from build123d import *

# Parameters (mm, degrees)
PAD_DEPTH         = 10
ARRAY001_COUNT    = 4
CYLINDER021_R     = 12
CYLINDER021_DEPTH = 124
CYLINDER022_R     = 22
CYLINDER022_DEPTH = 5
FILLET004_R       = 1
CYLINDER020_R     = 14
CYLINDER020_DEPTH = 124
FILLET001_R       = 0.6
FILLET002_R       = 1


with BuildPart() as long_hole_array:
    # Sketch → Pad (new body)
    with BuildSketch(Plane.XY):
        with BuildLine():
            ThreePointArc((-18.36954, -4), (-13.293607, -13.293607), (-4, -18.36954))
            ThreePointArc((-4, -18.36954), (-2.147351, -16.516891), (-4, -14.664242))
            ThreePointArc((-14.664242, -4), (-10.748023, -10.748023), (-4, -14.664242))
            ThreePointArc((-14.664242, -4), (-16.516891, -2.147351), (-18.36954, -4))
        make_face()
    extrude(amount=PAD_DEPTH)

    # Array001: long hole array ×4 about axis
    array001_axis = Axis((0, 0, 0), (0, 0, 1))


with BuildPart() as long_hole_array_1:
    add(long_hole_array.part)
    for i in range(1, ARRAY001_COUNT):
        add(long_hole_array.part.rotate(array001_axis, i * 360 / ARRAY001_COUNT))


with BuildPart() as top_hole_fusion:
    # Cylinder021 → Cylinder021 (new body)
    with BuildSketch(Plane.XY):
        Circle(CYLINDER021_R)
    extrude(amount=CYLINDER021_DEPTH)

    # Fusion004: union long hole array
    add(long_hole_array_1.part)


with BuildPart() as top_bottom_connector_fillet:
    # Cylinder022 → Cylinder022 (new body)
    with BuildSketch(Plane.XY):
        Circle(CYLINDER022_R)
    extrude(amount=CYLINDER022_DEPTH)

    # Fillet004
    fillet004_edges = [top_bottom_connector_fillet.edges().sort_by_distance(p)[0] for p in [
        (-22, 0, 5),
        (-22, 0, 0),
    ]]
    fillet(fillet004_edges, radius=FILLET004_R)


with BuildPart() as top_tube_cut_fillet:
    # Cylinder020 → Cylinder020 (new body)
    with BuildSketch(Plane.XY):
        Circle(CYLINDER020_R)
    extrude(amount=CYLINDER020_DEPTH)

    # Fillet001
    fillet001_edges = [top_tube_cut_fillet.edges().sort_by_distance(p)[0] for p in [
        (-14, 0, 124),
    ]]
    fillet(fillet001_edges, radius=FILLET001_R)

    # Fusion: union top bottom connector fillet
    add(top_bottom_connector_fillet.part)

    # Cut: cut top hole fusion
    add(top_hole_fusion.part, mode=Mode.SUBTRACT)

    # Fillet002
    fillet002_edges = [top_tube_cut_fillet.edges().sort_by_distance(p)[0] for p in [
        (-12, 0, 124),
    ]]
    fillet(fillet002_edges, radius=FILLET002_R)


solid = top_tube_cut_fillet.part
Geometry check sheet. Reference: the model listing, model coordinates, mm. A direction names the side the tool comes from. Round coordinates to 2 decimals unless told otherwise and drop trailing zeros. Order: outer loops, then holes, each group sorted by start corner. A loop starts at its lowest first (then second) coordinate and runs counter-clockwise, first axis right, second up. Notation, with made-up numbers: M -24,61 L 24,61 A11 cw 24,66 Z; hole C 83.5,29.25 d1. An arc over 180 degrees is marked long. Write each question's results on one line, items separated by ' | '. Start each with the question number.
1. Cross-section at A-A on x = 0. Record the boundary of the cut face in (y, z), plus the area to 3 significant figures.
2. Draft check along Y on faces 1 (the face through (12.932, -5.362, 63.371)), 2 (the face through (9, -9, 0)), 3 (the face through (2.148, -16.476, 2.465)). Enter one of: pulls with the +Y half, pulls with the -Y half, needs draft (parallel to the pull), parting line crosses it, or undercut.
3. Cross-section at C-C on z = 37.5. Record the boundary of the cut face in (x, y).
4. Cross-section at D-D on y = -6.5. Give the number of separate pieces and of enclosed holes in the cut face, plus the area to 3 significant figures.
5. Go/stop test with flat-tipped pins: P1, Ø8, axis at x = 1, z = 34.5, coming from the -Y side; P2, Ø14.5, axis at x = 0, y = 0, coming from the +Z side; P3, Ø5, axis at x = -3, y = 17.5, coming from the -Z side; P4, Ø8, axis at x = 14, z = 70, coming from the -Y side. Record where each tip stops, or that it passes through.
6. Set-up check for faces 4 (the face through (-13, 2, 124)), 5 (the face through (4, -14, 5)), 6 (the face through (-2.148, -16.558, 2.465)): record each of +Z, -Z, +X, -X, +Y, -Y from which the full face is reachable in a straight line by a thin tool's end or side.
7. Material ranges on L1, parallel to Y at x = 0, z = 97; L2, parallel to Y at x = -10, z = 104; L3, parallel to Z at x = 8.5, y = -17.5, recorded low to high. Write a range as from..to.
Resolved:
1) outline: M -22,1 A1 ccw -21,0 L -12,0 L -12,123 A1 ccw -13,124 L -13.4,124 A0.6 ccw -14,123.4 L -14,5 L -21,5 A1 ccw -22,4 Z; M 12,0 L 21,0 A1 ccw 22,1 L 22,4 A1 ccw 21,5 L 14,5 L 14,123.4 A0.6 ccw 13.4,124 L 13,124 A1 ccw 12,123 Z | area: 575 mm2
2) face 1: parting line crosses it | face 2: needs draft | face 3: undercut
3) outline: C 0,0 d28; hole C 0,0 d24
4) separate pieces: 4 | enclosed holes: 0 | area: 619 mm2
5) P1: y = -14 | P2: through | P3: z = 0 | P4: y = -9.8
6) face 4: +Z, +X, -X, +Y, -Y | face 5: +Z | face 6: +Z, -Z
7) L1: -14..-12, 12..14 | L2: -9.8..-6.63, 6.63..9.8 | L3: 0..5
